CAD build for the part. Positions are in the model's coordinates, mm. Face numbers are marked on the shaded views. A direction names the side the tool comes from. Round coordinates to 2 decimals unless told otherwise and drop trailing zeros. Loops run counter-clockwise (first coordinate to the right, second up) from the corner with the lowest first, then second, coordinate; pieces in that order, holes last.
Autodesk Inventor part; units mm, degrees
ref_plane "YZ Plane" through (0, 0, 0) normal (1, 0, 0) x (0, 1, 0)
ref_plane "XZ Plane" through (0, 0, 0) normal (0, 1, 0) x (-1, 0, 0)
ref_plane "XY Plane" through (0, 0, 0) normal (0, 0, 1) x (1, 0, 0)
sketch "Sketch1" plane through (0, 0, 0) normal (0, 0, 1) x (1, 0, 0)
  line L0 (-40, 40) -> (40, 40)
  line L1 (40, 40) -> (40, -40)
  line L2 (40, -40) -> (-40, -40)
  line L3 (-40, -40) -> (-40, 40)
  point P0 (0, 0)
  dimension "d0" = 80
  dimension "d1" = 80
  dimension "d2" = 40
  dimension "d3" = 40
extrude "Extrusion1" add sketch "Sketch1" against normal blind 15.9
sketch "Sketch2" plane through (0, 0, 0) normal (0, 0, 1) x (1, 0, 0)
  line L0 (0, 56) -> (0, -56)
  line L1 (-56, 0) -> (56, 0)
  point P0 (-20, 20)
  dimension "d6" = 20
  dimension "d7" = 20
hole "Hole1" at (-20, 20, 0) direction (0, 0, -1) diameter 8.4 end through all counterbore diameter 15 counterbore depth 8.9
mirror "Mirror1" about plane through (0, 0, 0) normal (1, 0, 0) of "Hole1"
mirror "Mirror2" about plane through (0, 0, 0) normal (0, 1, 0) of "Hole1", "Mirror1"
fillet "Fillet1" radius 3 4 edges at (-40, -40, -7.95) (-40, 40, -7.95) (40, 40, -7.95) (40, -40, -7.95)
properties part number "21-8000Z1" material "Aluminum-6061"
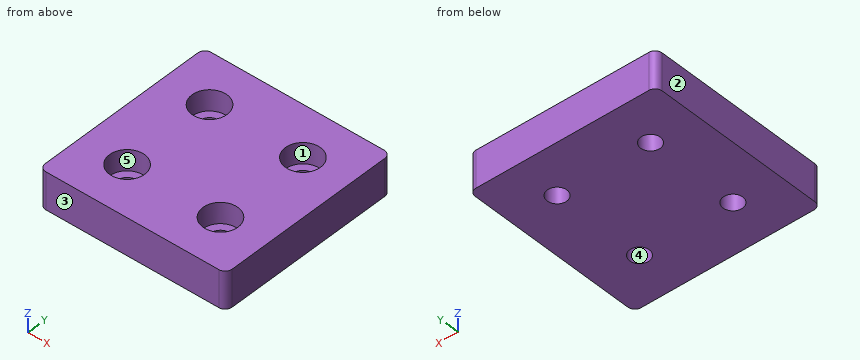
Item 1: Flat gauge pins, fed straight in: P1, Ø7.5, axis at x = 21.5, y = -20.5, coming from the +Z side; P2, Ø7.5, axis at x = 20, y = 20, coming from the -Z side; P3, Ø24, axis at x = -20, y = -20, coming from the -Z side. Where does each tip first touch, or does it go through?
Verdict:
P1: stops at z = -8.9
P2: passes through
P3: stops at z = -15.9
Item 2: Cut at B-B (z = -6). List the corners of the cut face in (x, y), plus the area to 3 significant figures.
Verdict:
outline: (-40, -37) arc R3 ccw to (-37, -40) - (37, -40) arc R3 ccw to (40, -37) - (40, 37) arc R3 ccw to (37, 40) - (-37, 40) arc R3 ccw to (-40, 37) - close; hole circle Ø15 at (-20, -20); hole circle Ø15 at (-20, 20); hole circle Ø15 at (20, -20); hole circle Ø15 at (20, 20)
area: 5,690 mm2
Item 3: 3-axis set-ups, long thin cutter, end or side, ignore diameter. For the marked faces 4 and 5: which of +Z, -Z, +X, -X, +Y, -Y reach the whole face in a straight line?
Verdict:
face 4: +Z, -Z
face 5: +Z
Item 4: Cut at A-A (y = -20). List the corners of the cut face in (x, z), plus the area to 3 significant figures.
Verdict:
outline: (-40, -15.9) - (-24.2, -15.9) - (-24.2, -8.9) - (-27.5, -8.9) - (-27.5, 0) - (-40, 0) - close; (-15.8, -15.9) - (15.8, -15.9) - (15.8, -8.9) - (12.5, -8.9) - (12.5, 0) - (-12.5, 0) - (-12.5, -8.9) - (-15.8, -8.9) - close; (24.2, -15.9) - (40, -15.9) - (40, 0) - (27.5, 0) - (27.5, -8.9) - (24.2, -8.9) - close
area: 887 mm2
Item 5: Wall check: L1, parallel to X at y = -20, z = -13.75; L2, parallel to X at y = -20, z = -1.75; L3, parallel to Y at x = -22, z = -8.75. Give the ranges that are in metal, low to high.
Verdict:
L1: x = -40 to -24.2, -15.8 to 15.8, 24.2 to 40
L2: x = -40 to -27.5, -12.5 to 12.5, 27.5 to 40
L3: y = -40 to -27.23, -12.77 to 12.77, 27.23 to 40
Item 6: Mould opens along Y. For the marked faces 1, 2 and 3 say: released by +Y, released by -Y, zero draft, split by the parting line, or undercut.
Verdict:
face 1: undercut
face 2: zero draft
face 3: released by -Y
Item 7: Cut at D-D (x = 26). List the corners of the cut face in (y, z), plus the area to 3 significant figures.
Verdict:
outline: (-40, -15.9) - (40, -15.9) - (40, 0) - (24.5, 0) - (24.5, -8.9) - (15.5, -8.9) - (15.5, 0) - (-15.5, 0) - (-15.5, -8.9) - (-24.5, -8.9) - (-24.5, 0) - (-40, 0) - close
area: 1,110 mm2
